Work out the finished part from the listing and answer in its coordinate system (mm). A direction names the side the tool comes from. Give positions to 0.01 mm unless a question says otherwise; leave off trailing zeros. Order: outer loops, then holes, each group sorted by start corner. A loop starts at its lowest first (then second) coordinate and runs counter-clockwise, first axis right, second up. Notation, with made-up numbers: M 38,34.5 L 84,34.5 A16 ccw 84,57.5 Z; hole C 75.25,42 d2. An arc over 180 degrees is marked long. One line per item, written item: value.
from build123d import *

# Parameters (mm, degrees)
SKETCH1_R            = 127
BOSS_EXTRUDE1_DEPTH  = 3.175
M3_CLEARANCE_HOLE1_D = 3.4
CIRPATTERN1_COUNT    = 8
BOSS_EXTRUDE2_DEPTH  = 3.175
CIRPATTERN2_COUNT    = 8
CUT_EXTRUDE1_REACH   = 266.384


with BuildPart() as part:
    # Sketch1 → Boss-Extrude1 (new body)
    with BuildSketch(Plane.XY):
        Circle(SKETCH1_R)
    extrude(amount=BOSS_EXTRUDE1_DEPTH)

    # M3 Clearance Hole1 (through all)
    with Locations(Plane(origin=(0, 0, 0), x_dir=(-1, 0, 0), z_dir=(0, 0, -1))):
        with Locations((-58.2494214, 58.493652703), (-82.549819355, -0.172697611), (-93.238867767, 66.113565457), (-112.679186132, 19.180485205), (-11.733270063, 4.860079591), (-68.767621753, 45.667457762), (-80.917820731, 16.334282605), (-35.199810189, 14.580238773)):
            m3_clearance_hole1 = Hole(M3_CLEARANCE_HOLE1_D / 2)

    # CirPattern1: M3 Clearance Hole1 ×8 about axis
    cirpattern1_axis = Axis((-0.09749486, -0.040383693, 0), (0, 0, 1))
    for i in range(1, CIRPATTERN1_COUNT):
        add(m3_clearance_hole1.rotate(cirpattern1_axis, i * 360 / CIRPATTERN1_COUNT), mode=Mode.SUBTRACT)

    # Sketch6 → Boss-Extrude2 (add)
    with BuildSketch(Plane(origin=(0, 0, 0), x_dir=(-1, 0, 0), z_dir=(0, 0, -1))):
        with BuildLine():
            Line((-100.530886518, 72.570613756), (-138.664014222, 88.365872427))
            ThreePointArc((-138.664014222, 88.365872427), (-160.534372382, 88.365872427), (-175.999050943, 72.901193866))
            Line((-175.999050943, 72.901193866), (-186.934230023, 46.501336224))
            Line((-186.934230023, 46.501336224), (-122.401244677, 19.770898473))
            Line((-122.401244677, 19.770898473), (-100.530886518, 72.570613756))
        make_face()
    boss_extrude2 = extrude(amount=-BOSS_EXTRUDE2_DEPTH)

    # CirPattern2: Boss-Extrude2 ×8 about axis
    cirpattern2_axis = Axis((0, 0, 0), (0, 0, 1))
    for i in range(1, CIRPATTERN2_COUNT):
        add(boss_extrude2.rotate(cirpattern2_axis, i * 360 / CIRPATTERN2_COUNT))

    # Sketch8 → Cut-Extrude1 (cut, up to next)
    with BuildSketch(Plane(origin=(0, 0, 0), x_dir=(-1, 0, 0), z_dir=(0, 0, -1)), mode=Mode.PRIVATE) as cut_extrude1_sk1:
        Polygon((-6.774206629, 2.80596826), (-5.81714311, -4.463650901), (0.957063519, -7.269619162), (6.774206629, -2.80596826), (5.81714311, 4.463650901), (-0.957063519, 7.269619162), align=None)
    cut_extrude1_tool1 = extrude(cut_extrude1_sk1.sketch, amount=-CUT_EXTRUDE1_REACH, mode=Mode.PRIVATE) & part.part
    add(cut_extrude1_tool1.solids().sort_by_distance((0, 0, 0))[0], mode=Mode.SUBTRACT)


solid = part.part
(1) Section C-C, the plane x = 119.5 is taken. Give the vertices of the cut face in (y, z) (3 decimals).
Findings:
outline: M -80.428,0 L 80.428,0 L 80.428,3.175 L -80.428,3.175 Z
(2) Determine the mould class of faces 1 (the cylindrical face through (90.011, 89.594, 1.565)), 2 (the flat face through (134.658, -86.707, 1.565)), 3 (the flat face through (-33.907, 156.529, 1.565)) for opening direction Y: pulls with the +Y half, pulls with the -Y half, needs draft (parallel to the pull), parting line crosses it, or undercut.
Findings:
face 1: undercut
face 2: pulls with the -Y half
face 3: pulls with the +Y half
(3) Section D-D, the plane y = -120.5 is taken. Give the vertices of the cut face in (x, z) (3 decimals).
Findings:
outline: M -80.842,0 L 80.842,0 L 80.842,3.175 L -80.842,3.175 Z
(4) Section B-B, the plane z = 2.15 is taken. Give the number of separate pieces and of enclosed holes in the cut face, then the cut area to 3 significant figures.
Findings:
separate pieces: 1
enclosed holes: 57
area: 78,100 mm^2
(5) Given P1, Ø5.5, axis at x = -112.87, y = 19.18, coming from the +Z side (3 decimals); P2, Ø1.5, axis at y = 97, z = 1, coming from the +X side; P3, Ø1, axis at y = -63.5, z = 1, coming from the +X side, each flat-ended and moving along its own axis, determine where each tip first touches the part or whether it passes through.
Findings:
P1: stops at z = 3.175
P2: stops at x = 82.85
P3: stops at x = 178.16
(6) Section A-A, the plane y = 156 is taken. Give the vertices of the cut face in (x, z) (3 decimals).
Findings:
outline: M -89.815,0 L -33.688,0 L -33.688,3.175 L -89.815,3.175 Z; M 33.688,0 L 95.547,0 L 95.547,3.175 L 33.688,3.175 Z
(7) Which of the six approach directions +Z, -Z, +X, -X, +Y, -Y give full straight-line access (tool end or side, diameter ignored) to faces 4 (the flat face through (28.16, 142.65, 1.57)), 5 (the flat face through (156.529, 33.907, 1.565)), 6 (the flat face through (-156.529, -33.907, 1.565))?
Findings:
face 4: +Z, -Z, +Y
face 5: +Z, -Z, +X
face 6: +Z, -Z, -X
(8) Find the intervals of material crossed by probe 1 along Y at (x, z) = (-82, 0.55); probe 2 along X at (y, z) = (4, 2.6); probe 3 along Y at (x, z) = (-18, 0.8), in increasing order. Write a range as from..to.
Findings:
probe 1: y = -172.23..-123.3, -96.98..-17.87, -14.96..-1.7, 1.62..14.88, 17.78..96.98, 123.3..169.97
probe 2: x = -126.94..-13.39, -10.46..-5.88, 5.22..10.27, 13.2..126.94
probe 3: y = -125.72..-113.89, -111.74..-81.8, -80.31..80.23, 81.72..111.66, 113.81..125.72
